Can you work these out from the model? Positions are in its coordinate system, mm. A direction names the side the tool comes from. Give positions to 0.01 mm unless a question says otherwise; leave off trailing zeros. Order: outer loops, then holes, each group sorted by start corner. A loop starts at its lowest first (then second) coordinate and runs counter-clockwise, first axis right, second up. Notation, with made-up numbers: (-1, -8.75) - (11, -8.75) arc R18 cw to (11, 11.25) - close; hole circle Ø9 at (27.25, -35.75). An arc over 180 degrees is marked (long way). Return JSON: item names as keys, results as strings.
```python
from build123d import *

# Parameters (mm, degrees)
SKETCH_1_W          = 120
SKETCH_1_H          = 120
EXTRUDE_1_DEPTH     = 52
SKETCH_2_W          = 96
SKETCH_2_H          = 50
CUT_EXTRUDE_1_DEPTH = 144.888845989
SKETCH_4_W          = 10
SKETCH_4_H          = 50
CUT_EXTRUDE_2_DEPTH = 144.888845989
SKETCH_5_W          = 10
SKETCH_5_H          = 50
CUT_EXTRUDE_3_DEPTH = 144.888845989
FILLET_1_R          = 2


with BuildPart() as part:
    # 草图1 → 凸台-拉伸1 (new body)
    with BuildSketch(Plane(origin=(0, 52, 0), x_dir=(1, 0, 0), z_dir=(0, 1, 0))):
        Rectangle(SKETCH_1_W, SKETCH_1_H)
    extrude(amount=-EXTRUDE_1_DEPTH)

    # 草图2 → 切除-拉伸1 (cut, through all)
    with BuildSketch(Plane(origin=(0, 0, -60), x_dir=(-1, 0, 0), z_dir=(0, 0, -1))):
        with Locations((0, 27)):
            Rectangle(SKETCH_2_W, SKETCH_2_H)
    extrude(amount=-CUT_EXTRUDE_1_DEPTH, mode=Mode.SUBTRACT)

    # 草图4 → 切除-拉伸2 (cut, through all)
    with BuildSketch(Plane.XY.offset(60)):
        with Locations((55, 25)):
            Rectangle(SKETCH_4_W, SKETCH_4_H)
    extrude(amount=-CUT_EXTRUDE_2_DEPTH, mode=Mode.SUBTRACT)

    # 草图5 → 切除-拉伸3 (cut, through all)
    with BuildSketch(Plane(origin=(0, 0, -60), x_dir=(-1, 0, 0), z_dir=(0, 0, -1))):
        with Locations((55, 25)):
            Rectangle(SKETCH_5_W, SKETCH_5_H)
    extrude(amount=-CUT_EXTRUDE_3_DEPTH, mode=Mode.SUBTRACT)

    # 圆角1
    fillet_1_edges = [part.edges().sort_by_distance(p)[0] for p in [
        (48, 52, 0),
        (-48, 52, 0),
        (50, 0, 0),
        (-50, 0, 0),
    ]]
    fillet(fillet_1_edges, radius=FILLET_1_R)


solid = part.part
```
1. If I drill on L1, parallel to X at y = 24, z = -27.5; L2, parallel to Y at x = -40, z = 33.5, over which ranges is the centre line in solid material (lowest first)? Write a range as [from, to].
Checks:
{"L1": "[-50, -48], [48, 50]", "L2": "[0, 2]"}
2. Suppose I cut it at A-A (y = 18). List the corners of the cut face in (x, z) for me.
Checks:
{"outline": "(-50, -60) - (-48, -60) - (-48, 60) - (-50, 60) - close; (48, -60) - (50, -60) - (50, 60) - (48, 60) - close"}
3. Suppose I cut it at C-C (x = -26.5). List the corners of the cut face in (y, z) for me.
Checks:
{"outline": "(0, -60) - (2, -60) - (2, 60) - (0, 60) - close"}
4. Thinking about a two-plate mould opening in X: for faces 1 (the face through (1, 2, -1)), 2 (the face through (-50, 26, -1)), 3 (the face through (-48, 26, -1)), 4 (the face through (55, 52, -1)), which applies, +X half, -X half, draft (parallel to the pull), parting line (faces both ways), or undercut?
Checks:
{"face 1": "undercut", "face 2": "-X half", "face 3": "undercut", "face 4": "draft"}
5. Suppose I cut it at B-B (z = 25.5). List the corners of the cut face in (x, y) for me.
Checks:
{"outline": "(-60, 50) - (-50, 50) - (-50, 2) arc R2 ccw to (-48, 0) - (48, 0) arc R2 ccw to (50, 2) - (50, 50) - (60, 50) - (60, 52) - (50, 52) arc R2 ccw to (48, 50) - (48, 2) - (-48, 2) - (-48, 50) arc R2 ccw to (-50, 52) - (-60, 52) - close"}
6. On a 3-axis mill with a long thin cutter (end or side, diameter ignored), from which of +Z, -Z, +X, -X, +Y, -Y can I reach the whole of each face in a straight line? I mean faces 5 (the face through (48, 26, -1)), 6 (the face through (-55, 50, -1)), 7 (the face through (50, 26, 1)). Say none if no direction works.
Checks:
{"face 5": "+Z, -Z, +Y", "face 6": "+Z, -Z, -X, -Y", "face 7": "+Z, -Z, +X, -Y"}
7. For pin 1 Ø11 at (x, z) = (-56.5, 20) entering from -Y; pin 2 Ø8 at (y, z) = (34, 18.5) entering from -X; pin 3 Ø8 at (y, z) = (22, -36.5) entering from +X; pin 4 Ø8 at (x, y) = (27.5, 8.5) entering from -Z, each with a flat end and sliding along its axis, tell me the tip position at first contact or that it passes through.
Checks:
{"pin 1": "y = 50", "pin 2": "x = -50", "pin 3": "x = 50", "pin 4": "through"}
